```python
from build123d import *

# Parameters (mm, degrees)
BOSS_EXTRUDE1_DEPTH  = 10
FILLET1_R            = 5
SKETCH2_R            = 12.5
BOSS_EXTRUDE2_DEPTH  = 20
SKETCH3_R            = 12.5
BOSS_EXTRUDE3_DEPTH  = 50
FILLET1_OF_MIRROR1_R = 5


with BuildPart() as part:
    # Sketch1 → Boss-Extrude1 (new body)
    with BuildSketch(Plane.XY):
        with BuildLine():
            Line((-17.5, 30), (-22.789809421, 0))
            Line((-22.789809421, 0), (-50, 0))
            ThreePointArc((-50, 0), (0, -50), (50, 0))
            Line((50, 0), (22.789809421, 0))
            Line((22.789809421, 0), (17.5, 30))
            ThreePointArc((17.5, 30), (0, 47.5), (-17.5, 30))
        make_face()
    boss_extrude1 = extrude(amount=-BOSS_EXTRUDE1_DEPTH)

    # Fillet1
    fillet1_edges = [part.edges().sort_by_distance(p)[0] for p in [
        (-50, 0, -5),
        (-22.789809421, 0, -5),
        (-17.5, 30, -5),
        (17.5, 30, -5),
        (22.789809421, 0, -5),
        (50, 0, -5),
    ]]
    fillet(fillet1_edges, radius=FILLET1_R)

    # Sketch2 → Boss-Extrude2 (add)
    with BuildSketch(Plane.XY):
        Circle(SKETCH2_R)
    boss_extrude2 = extrude(amount=BOSS_EXTRUDE2_DEPTH)

    # Sketch3 → Boss-Extrude3 (add)
    with BuildSketch(Plane(origin=(0, 0, -10), x_dir=(-1, 0, 0), z_dir=(0, 0, -1))):
        with Locations(Location((0, 30, 0), (0, 0, 180))):
            Circle(SKETCH3_R)
    extrude(amount=BOSS_EXTRUDE3_DEPTH)

    # Mirror1: Boss-Extrude1, Boss-Extrude2 across plane
    add(boss_extrude1.mirror(Plane(origin=(0, 0, -35), x_dir=(1, 0, 0), z_dir=(0, 0, -1))))
    add(boss_extrude2.mirror(Plane(origin=(0, 0, -35), x_dir=(1, 0, 0), z_dir=(0, 0, -1))))

    # Fillet1 of Mirror1
    fillet1_of_mirror1_edges = [part.edges().sort_by_distance(p)[0] for p in [
        (-50, 0, -65),
        (-22.789809421, 0, -65),
        (-17.5, 30, -65),
        (17.5, 30, -65),
        (22.789809421, 0, -65),
        (50, 0, -65),
    ]]
    fillet(fillet1_of_mirror1_edges, radius=FILLET1_OF_MIRROR1_R)


solid = part.part
```
Here's how the part is built. I have some questions about the finished solid (model axes, mm). A direction names the side the tool comes from. Give positions to 0.01 mm unless a question says otherwise; leave off trailing zeros. Loops run counter-clockwise (first coordinate to the right, second up) from the corner with the lowest first, then second, coordinate; pieces in that order, holes last. Notation, with made-up numbers: M 78.5,75.25 L 100.5,75.25 A10 cw 100.5,82.25 Z; hole C -6.5,62 d2. An arc over 180 degrees is marked long. Put each result on its own line as item: value. Start each with the question number.
(1) I want a section at B-B on x = -35. Please give me the cut outline in (y, z), then the cut area to 3 significant figures.
(2) I want a section at C-C on x = 0. Please give me the cut outline in (y, z), then the cut area to 3 significant figures.
(3) For faces 5 (the cylindrical face through (11.923, 3.755, 9.86)), 6 (the cylindrical face through (11.923, 3.755, -79.86)), 7 (the flat face through (36, 0, -5)), which set-ups out of +Z, -Z, +X, -X, +Y, -Y let a thin tool reach every point of the face, with its end or its side?
(4) I want a section at D-D on z = -29.5. Please give me the cut outline in (x, y), then the cut area to 3 significant figures.
(5) I want a section at A-A on y = -9. Please give me the cut outline in (x, z).
(6) If we mould it in two halves opening along Z, with no side actions, what happens to faces 1 (the cylindrical face through (-48.409, -1.623, -5.07)), 2 (the cylindrical face through (-2.71, 42.203, -34.65)), 3 (the flat face through (0, 0, 20)), 4 (the flat face through (-1, -11, -60))? For each: +Z half, -Z half, draft (parallel to the pull), parting line (faces both ways), or undercut.
(7) I need wall thicknesses on line 1 along Z through (x, y) = (-14, -8.5); line 2 along Z through (x, y) = (-3, 20.5); line 3 along Y through (x, z) = (-4.5, -84.5). Which ranges of each line are inside material? Lowest first, please. Write a range as [from, to].
(8) Will these pins go through, and if not, where does the flat tip stop? pin 1 Ø8 at (x, z) = (39, -6.5) entering from +Y; pin 2 Ø6 at (x, y) = (36.5, -8.5) entering from -Z; pin 3 Ø6 at (x, z) = (-5.5, -66.5) entering from +Y.
Answer block:
1. outline: M -35.71,-70 L 0,-70 L 0,-60 L -35.71,-60 Z; M -35.71,-10 L 0,-10 L 0,0 L -35.71,0 Z
1. area: 714 mm^2
2. outline: M -50,-70 L -12.5,-70 L -12.5,-90 L 12.5,-90 L 12.5,-70 L 47.5,-70 L 47.5,-60 L 42.5,-60 L 42.5,-10 L 47.5,-10 L 47.5,0 L 12.5,0 L 12.5,20 L -12.5,20 L -12.5,0 L -50,0 L -50,-10 L 17.5,-10 L 17.5,-60 L -50,-60 Z
2. area: 4,200 mm^2
3. face 5: +Z
3. face 6: -Z
3. face 7: +Z, -Z, +X, +Y
4. outline: C 0,30 d25
4. area: 491 mm^2
5. outline: M -49.18,-70 L -8.67,-70 L -8.67,-90 L 8.67,-90 L 8.67,-70 L 49.18,-70 L 49.18,-60 L -49.18,-60 Z; M -49.18,-10 L 49.18,-10 L 49.18,0 L 8.67,0 L 8.67,20 L -8.67,20 L -8.67,0 L -49.18,0 Z
6. face 1: draft
6. face 2: undercut
6. face 3: +Z half
6. face 4: undercut
7. line 1: [-70, -60], [-10, 0]
7. line 2: [-70, 0]
7. line 3: [-11.66, 11.66]
8. pin 1: y = 0
8. pin 2: z = -70
8. pin 3: y = 47.32
